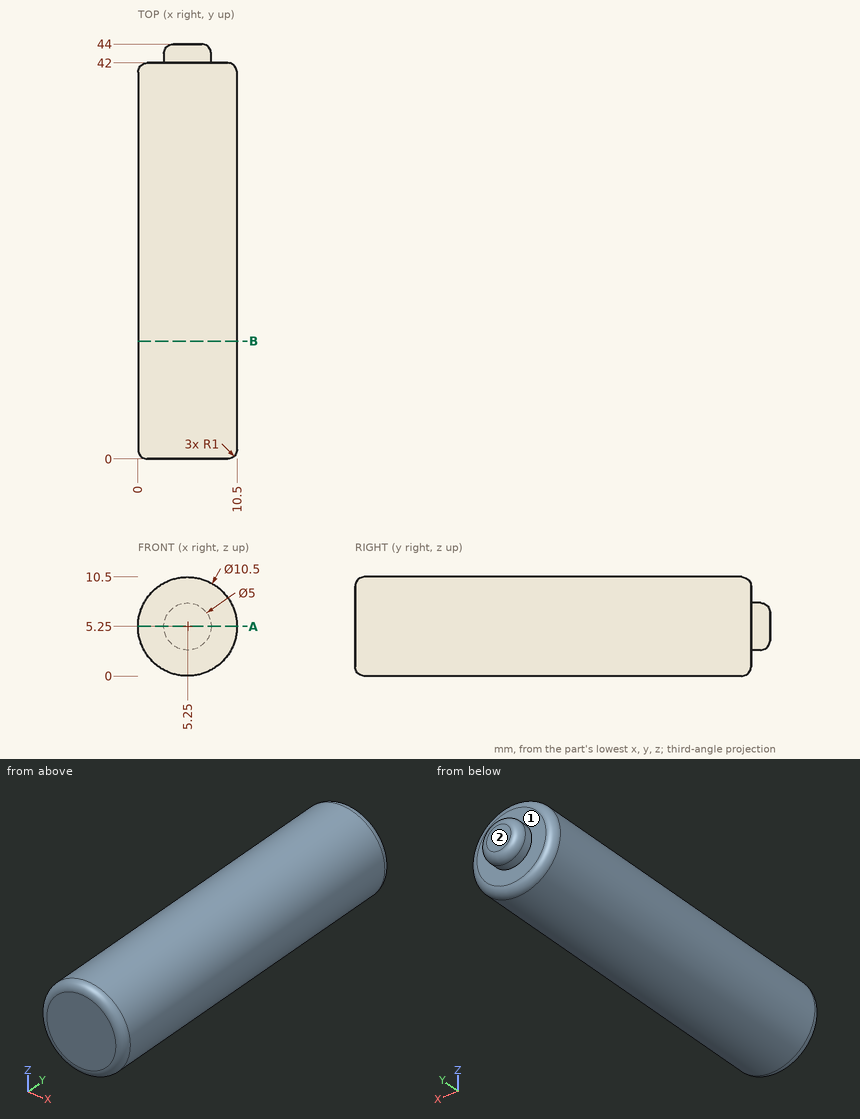
The drawing under review shows one solid part. Ordinate dimensions are in mm from its lowest x, y, z. A direction names the side the tool comes from. Coordinates: 2 decimals unless noted, no trailing zeros. Write each loop counter-clockwise with the first axis right and the second up, starting at its lowest first coordinate (ties: lowest second). Pieces come first, ordered by that corner, then holes. Notation, with made-up numbers: (-24.5, -9) - (2.5, -9) arc R21 cw to (2.5, 11) - close; hole circle Ø1 at (21.5, 14). An arc over 180 degrees is marked (long way). Put each result on its own line as item: value.
1. Add section B-B, the plane y = 12.5. Give the boundary of the cut face in (x, z), then the cut area to 3 significant figures.
Values found:
outline: circle Ø10.5 at (5.25, 5.25)
area: 86.6 mm²
2. For pin 1 (3 mm diameter, centred on x = 2.5, y = 36, fed in from +Z); pin 2 (3 mm diameter, centred on y = 13.5, z = 8, fed in from -X); pin 3 (5 mm diameter, centred on y = 13.5, z = 9, fed in from +X), all flat-tipped, find the tip position at first contact; note any pin that passes through.
Values found:
pin 1: z = 10.35
pin 2: x = 0.15
pin 3: x = 10.35
3. Add section A-A, the plane z = 5.25. Give the boundary of the cut face in (x, y), then the cut area to 3 significant figures.
Values found:
outline: (0, 1) arc R1 ccw to (1, 0) - (9.5, 0) arc R1 ccw to (10.5, 1) - (10.5, 41) arc R1 ccw to (9.5, 42) - (7.75, 42) - (7.75, 43) arc R1 ccw to (6.75, 44) - (3.75, 44) arc R1 ccw to (2.75, 43) - (2.75, 42) - (1, 42) arc R1 ccw to (0, 41) - close
area: 450 mm²
4. Machinability: for the marked faces 1 and 2, which of the approach directions +Z, -Z, +X, -X, +Y, -Y give a long, thin tool a straight path to every point of the face, cutting with its end or side? Answer none if there is none.
Values found:
face 1: +Y
face 2: +Z, -Z, +X, -X, +Y
5. Wall thickness on probe 1 along Y at (x, z) = (7.75, 8.75); probe 2 along Z at (x, y) = (6.5, 31); probe 3 along Z at (x, y) = (5.5, 33): over which ranges is each line inside the solid? List them lowest first.
Values found:
probe 1: 0 to 42
probe 2: 0.15 to 10.35
probe 3: 0.01 to 10.49
